Job drawing, mm, ordinate dimensions from the low corner. One solid piece. A direction names the side the tool comes from. Give positions to 0.01 mm unless a question says otherwise; leave off trailing zeros. Write each loop counter-clockwise with the first axis right and the second up, starting at its lowest first coordinate (ties: lowest second). Pieces come first, ordered by that corner, then holes. Notation, with made-up numbers: (-21, 24.5) - (7, 24.5) arc R7 cw to (7, 34.5) - close; hole circle Ø4 at (57.5, -38). An arc over 180 degrees is marked (long way). Answer in a Markdown table with one row per item. Add a question column.
1. Pull direction Y, two halves, no side cores. Call the marked faces 3, 4 and 5: released by +Y, released by -Y, zero draft, split by the parting line, or undercut.
2. Band-saw the part on D-D on z = 18.75. Write the cut outline in (x, y), plus the area to 3 significant figures.
3. Band-saw the part on A-A on x = 20. Write the cut outline in (y, z).
4. Drop flat-ended pins along their axis: pin 1 Ø3 at (x, z) = (16, 3) entering from +Y; pin 2 Ø9 at (x, z) = (6.5, 10) entering from -Y; pin 3 Ø8 at (y, z) = (9.5, 9.5) entering from +X; pin 4 Ø10 at (x, z) = (16, 13.5) entering from +Y. Give the stop position or say it passes through.
5. Band-saw the part on B-B on z = 5.75. Write the cut outline in (x, y), plus the area to 3 significant figures.
6. Band-saw the part on C-C on x = 6.5. Write the cut outline in (y, z), plus the area to 3 significant figures.
7. Probe line 1 along Y through (x, z) = (20, 2); line 2 along X through (y, z) = (9, 3.75); line 3 along X through (y, z) = (0.75, 9.25). List the from-to ranges inside material, lowest first.
8. Which spindle directions (+Z, -Z, +X, -X, +Y, -Y) get a long thin tool onto all of the face, cutting with end or side? Do the marked faces 1 and 2. Say none if no direction does.
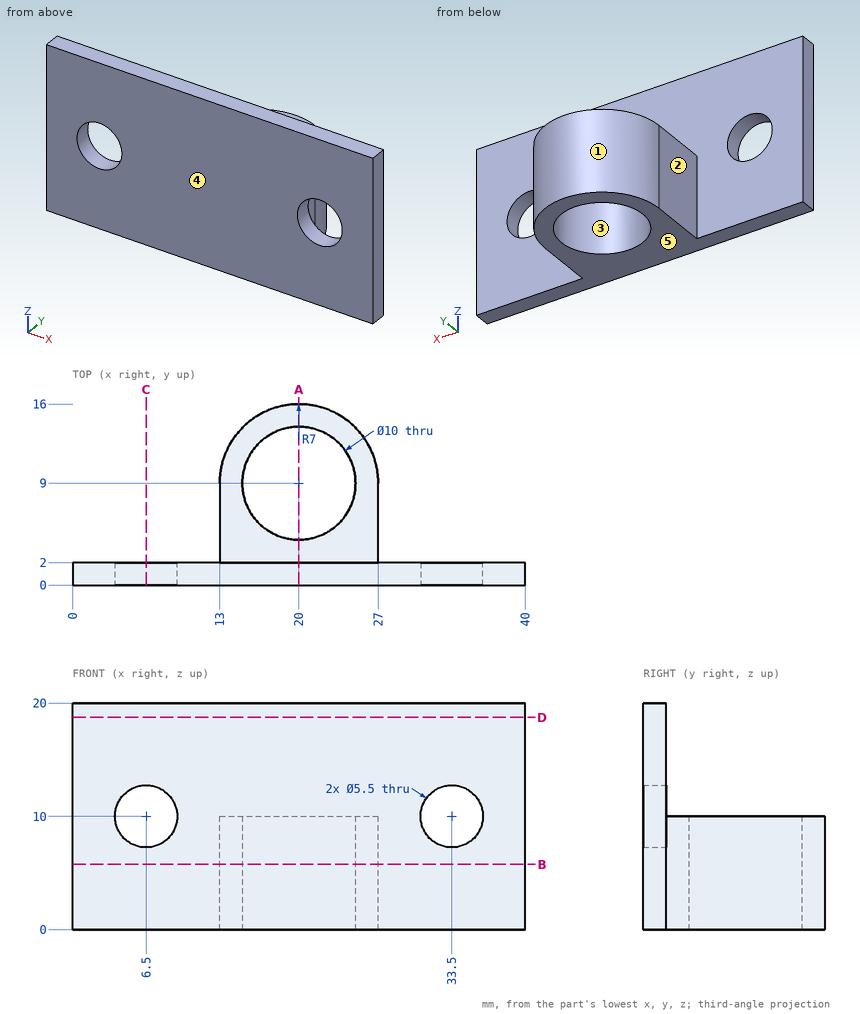
Values:
| question | item | result |
|---|---|---|
| 1 | face 3 | undercut |
| 1 | face 4 | released by -Y |
| 1 | face 5 | zero draft |
| 2 | outline | (0, 0) - (40, 0) - (40, 2) - (0, 2) - close |
| 2 | area | 80.0 mm² |
| 3 | outline | (0, 0) - (4, 0) - (4, 10) - (2, 10) - (2, 20) - (0, 20) - close; (14, 0) - (16, 0) - (16, 10) - (14, 10) - close |
| 4 | pin 1 | stops at y = 15.54 |
| 4 | pin 2 | stops at y = 0 |
| 4 | pin 3 | stops at x = 27 |
| 4 | pin 4 | stops at y = 15.99 |
| 5 | outline | (0, 0) - (40, 0) - (40, 2) - (27, 2) - (27, 9) arc R7 ccw to (13, 9) - (13, 2) - (0, 2) - close; hole circle Ø10 at (20, 9) |
| 5 | area | 176 mm² |
| 6 | outline | (0, 0) - (2, 0) - (2, 7.25) - (0, 7.25) - close; (0, 12.75) - (2, 12.75) - (2, 20) - (0, 20) - close |
| 6 | area | 29.0 mm² |
| 7 | line 1 | y = 0 to 4, 14 to 16 |
| 7 | line 2 | x = 13 to 15, 25 to 27 |
| 7 | line 3 | x = 0 to 3.85, 9.15 to 30.85, 36.15 to 40 |
| 8 | face 1 | +Z, -Z, +Y |
| 8 | face 2 | +Z, -Z, -X, +Y |
